Work out the finished part from the listing and answer in its coordinate system (mm). A direction names the side the tool comes from. Give positions to 0.01 mm unless a question says otherwise; leave off trailing zeros. Order: outer loops, then holes, each group sorted by start corner. A loop starts at its lowest first (then second) coordinate and runs counter-clockwise, first axis right, second up.
```python
from build123d import *

# Parameters (mm, degrees)
SKETCH1_W               = 50.8
SKETCH1_H               = 25.4
BOSS_EXTRUDE1_DEPTH     = 381
SHELL1_T                = -3.175
SKETCH4_R               = 2.38125
CUT_EXTRUDE1_DEPTH      = 385.581499815
CUT_EXTRUDE2_DEPTH      = 383.689587002
CUT_EXTRUDE2_DEPTH_BACK = 383.689587002
SKETCH5_R               = 2.38125


with BuildPart() as part:
    # Sketch1 → Boss-Extrude1 (new, symmetric)
    with BuildSketch(Plane(origin=(0, 0, 0), x_dir=(1, 0, 0), z_dir=(0, 1, 0))):
        Rectangle(SKETCH1_W, SKETCH1_H)
    extrude(amount=BOSS_EXTRUDE1_DEPTH, both=True)

    # Shell1
    shell1_openings = [part.faces().sort_by_distance(p)[0] for p in [
        (0, 381, 0),
        (0, -381, 0),
    ]]
    offset(amount=SHELL1_T, openings=shell1_openings, kind=Kind.INTERSECTION)

    # Sketch4 → Cut-Extrude1 (cut, through all)
    with BuildSketch(Plane(origin=(25.4, 0, 0), x_dir=(0, 0, -1), z_dir=(1, 0, 0))):
        with Locations((0, 110.9345)):
            Circle(SKETCH4_R)
        with Locations((0, 98.2345)):
            Circle(SKETCH4_R)
        with Locations((0, 85.5345)):
            Circle(SKETCH4_R)
        with Locations(Location((0, -85.5345, 0), (0, 0, 180))):
            Circle(SKETCH4_R)
        with Locations(Location((0, -98.2345, 0), (0, 0, 180))):
            Circle(SKETCH4_R)
        with Locations(Location((0, -110.9345, 0), (0, 0, 180))):
            Circle(SKETCH4_R)
    extrude(amount=-CUT_EXTRUDE1_DEPTH, mode=Mode.SUBTRACT)

    # Sketch5 → Cut-Extrude2 (cut, two sides: drawn at the far end of the back side and taken through both)
    with BuildSketch(Plane.XY.offset(12.7).offset(-CUT_EXTRUDE2_DEPTH_BACK)):
        with Locations((-12.7, 368.3)):
            Circle(SKETCH5_R)
        with Locations((12.7, 368.3)):
            Circle(SKETCH5_R)
        with Locations((12.7, 342.9)):
            Circle(SKETCH5_R)
        with Locations((-12.7, 342.9)):
            Circle(SKETCH5_R)
        with Locations((-12.7, -342.9)):
            Circle(SKETCH5_R)
        with Locations((12.7, -342.9)):
            Circle(SKETCH5_R)
        with Locations((12.7, -368.3)):
            Circle(SKETCH5_R)
        with Locations((-12.7, -368.3)):
            Circle(SKETCH5_R)
    extrude(amount=CUT_EXTRUDE2_DEPTH + CUT_EXTRUDE2_DEPTH_BACK, mode=Mode.SUBTRACT)


solid = part.part
```
1. The part is cut by section A-A (x = -1). Write down the section's boundary in (y, z) (3 decimals), then the cut area to 3 significant figures.
Findings below:
outline: (-381, -12.7) - (381, -12.7) - (381, -9.525) - (-381, -9.525) - close; (-381, 9.525) - (381, 9.525) - (381, 12.7) - (-381, 12.7) - close
area: 4,840 mm2
2. The part is cut by section B-B (y = -139.5). Write down the section's boundary in (x, z) (3 decimals).
Findings below:
outline: (-25.4, -12.7) - (25.4, -12.7) - (25.4, 12.7) - (-25.4, 12.7) - close; hole (-22.225, -9.525) - (22.225, -9.525) - (22.225, 9.525) - (-22.225, 9.525) - close
3. Straight lines are drawn through the part: probe 1 along X at (y, z) = (368.3, 11.1); probe 2 along Y at (x, z) = (-12.7, 11.95); probe 3 along Z at (x, y) = (-14.5, -239) (3 decimals). For each, find the intervals that lie inside material, in ascending order.
Findings below:
probe 1: x = -25.4 to -15.08, -10.32 to 10.32, 15.08 to 25.4
probe 2: y = -381 to -370.68, -365.92 to -345.28, -340.52 to 340.52, 345.28 to 365.92, 370.68 to 381
probe 3: z = -12.7 to -9.525, 9.525 to 12.7
4. The mould has two halves that part along X. Classify faces 3 (the face through (25.4, 5, 0)), 4 (the face through (22.225, 5, 0)), 5 (the face through (-25.4, 5, 0)): pulls with the +X half, pulls with the -X half, needs draft (parallel to the pull), parting line crosses it, or undercut.
Findings below:
face 3: pulls with the +X half
face 4: undercut
face 5: pulls with the -X half
5. Which of the six approach directions +Z, -Z, +X, -X, +Y, -Y give full straight-line access (tool end or side, diameter ignored) to faces 1 (the face through (0, -381, -10)), 2 (the face through (0, 5, 9.525))?
Findings below:
face 1: +Z, -Z, +X, -X, -Y
face 2: +Y, -Y
